The listing builds one solid part. Answer for the finished solid, in the listing's coordinates (mm). A direction names the side the tool comes from. Give positions to 0.01 mm unless a question says otherwise; leave off trailing zeros. Order: outer loops, then holes, each group sorted by start corner. A loop starts at its lowest first (then second) coordinate and runs counter-clockwise, first axis right, second up. Notation, with made-up numbers: (81.25, 53.5) - (138.25, 53.5) arc R11 ccw to (138.25, 67.5) - close; hole circle Ø4 at (39.5, 77.25). An arc over 180 degrees is marked (long way). Answer as a JSON object with one key per item and string values. Group by question number.
Q1. A cutting plane is placed at D-D, the plane x = 0.4. Give the vertices of the cut face in (y, z).
Q2. A cutting plane is placed at B-B, the plane x = 0. Give the vertices of the cut face in (y, z), and give its area (3 significant figures).
Q3. A cutting plane is placed at C-C, the plane z = -1. Give the vertices of the cut face in (x, y), and give its area (3 significant figures).
Q4. A cutting plane is placed at A-A, the plane x = 1.4. Give the vertices of the cut face in (y, z).
Q5. The mould has two halves that part along X. Classify faces 4 (the face through (-0.03, -1.14, -9.09)), 5 (the face through (-0.046, -2.538, -6.086)), 6 (the face through (-2, -3, -3)): released by +X, released by -X, zero draft, split by the parting line, or undercut.
Q6. For faces 1 (the face through (0, -3, -3.4)), 2 (the face through (-0.028, -1.185, -0.722)), 3 (the face through (-0.03, -2.17, -5.71)), determine the directions among +Z, -Z, +X, -X, +Y, -Y from which every point of the face is accessible in a straight line to the end or side of a thin tool.
Q7. Given pin 1 (1 mm diameter, centred on x = 0, y = -3, fed in from +Z); pin 2 (1 mm diameter, centred on x = 0.5, y = -4.5, fed in from -Z); pin 3 (1.5 mm diameter, centred on x = 1, y = -3.5, fed in from -Z), each flat-ended and moving along its own axis, determine where each tip first touches the part or whether it passes through.
Q8. Consider line 1 (Y direction, x = 0.25, z = -2); line 2 (Z direction, x = -1.45, y = -1.9); line 3 (X direction, y = -2.2, z = -7). Determine where each line is inside the solid, lowest interval first.
Autodesk Inventor part; units mm, degrees
ref_plane "YZ Plane" through (0, 0, 0) normal (1, 0, 0) x (0, 1, 0)
ref_plane "XZ Plane" through (0, 0, 0) normal (0, 1, 0) x (-1, 0, 0)
ref_plane "XY Plane" through (0, 0, 0) normal (0, 0, 1) x (1, 0, 0)
sketch "Skizze1" plane through (0, 0, 0) normal (1, 0, 0) x (0, 1, 0)
  line L0 (-1.5214, 0) -> (-5.9349, 0)
  line L1 (-5.9349, 0) -> (-1.5967, -9.3035)
  line L2 (0, -3.2627) -> (-1.5214, 0)
  line L3 (0, -3.2627) -> (-2.7189, -4.5306)
  line L4 (-2.7189, -4.5306) -> (-0.6904, -8.8808)
  line L5 (-0.6904, -8.8808) -> (-1.5967, -9.3035)
  line L6 (0, 1.8607) -> (0, -11.1642)
  point P0 (0, 0)
  dimension "d0" = 65
  dimension "d32" = 1
  dimension "d33" = 3
  dimension "d35" = 3.6
  dimension "d36" = 8.4
extrude "Extrusion1" add sketch "Skizze1" along normal mid plane 4
sketch "Skizze2" plane through (-2, -5.9349, 0) normal (0, 0, 1) x (1, 0, 0)
  line L0 (0, 0) -> (4, 0)
  line L1 (4, 4.4135) -> (4, 0)
  line L2 (4, 4.4135) -> (0, 4.4135)
  line L3 (0, 0) -> (0, 4.4135)
  line L4 (0, 4.3383) -> (0, 0) construction
  point P0 (2, 5.9349)
  point P1 (0, 4.7343)
  point P2 (2, 3.0135)
  dimension "d5" = 2
  dimension "d25" = 1.4
hole "Bohrung1" at (0, -2.9214, 0) direction (0, 0, -1) diameter 1.9 depth 3.4
sketch "Skizze3" plane through (-2, -1.8641, -8.7299) normal (0, -0.9063078, -0.4226183) x (1, 0, 0)
  line L0 (4, 9.6324) -> (4, -0.6329)
  line L1 (0, 9.6324) -> (4, 9.6324)
  line L2 (0, -0.6329) -> (0, 9.6324)
  line L3 (0, -0.6329) -> (4, -0.6329)
  point P0 (2, 1.6324)
  dimension "d26" = 2
  dimension "d29" = 8
hole "Bohrung2" at (0, -2.554, -7.2505) direction (0, 0.9063078, 0.4226183) diameter 2.1 end through all
chamfer "Fase1" distance 1.2 angle 45 1 edges at (0, 0, -3.2627)
fillet "Rundung1" radius 2 1 edges at (0, -0.5071, -2.1751)
properties part number "Ballsensor Platinenwinkel" material "PC/ABS-Kunststoff"
Reply:
{
 "1": {"outline": "(-5.93, 0) - (-2.96, -6.37) - (-2.06, -5.95) - (-2.72, -4.53) - (-1.09, -3.77) - (-0.79, -2.95) arc R2 ccw to (-0.86, -1.42) - (-1.52, 0) - (-2.06, 0) - (-2.06, -3.4) - (-3.78, -3.4) - (-3.78, 0) - close; (-2.14, -8.13) - (-1.6, -9.3) - (-0.69, -8.88) - (-1.24, -7.71) - close"},
 "2": {"outline": "(-5.93, 0) - (-3, -6.3) - (-2.09, -5.88) - (-2.72, -4.53) - (-1.09, -3.77) - (-0.79, -2.95) arc R2 ccw to (-0.86, -1.42) - (-1.52, 0) - (-1.97, 0) - (-1.97, -3.4) - (-3.87, -3.4) - (-3.87, 0) - close; (-2.11, -8.2) - (-1.6, -9.3) - (-0.69, -8.88) - (-1.2, -7.78) - close", "area": "13.6 mm^2"},
 "3": {"outline": "(-2, -5.47) - (2, -5.47) - (2, -1.06) - (-2, -1.06) - close; hole circle Ø1.9 at (0, -2.92)", "area": "14.8 mm^2"},
 "4": {"outline": "(-5.93, 0) - (-1.6, -9.3) - (-0.69, -8.88) - (-2.72, -4.53) - (-1.09, -3.77) - (-0.79, -2.95) arc R2 ccw to (-0.86, -1.42) - (-1.52, 0) - close"},
 "5": {"face 4": "zero draft", "face 5": "undercut", "face 6": "released by -X"},
 "6": {"face 1": "+Z", "face 2": "+Z, +X, -X, +Y", "face 3": "+X, -X, +Y"},
 "7": {"pin 1": "stops at z = -3.4", "pin 2": "stops at z = -4.15", "pin 3": "stops at z = -6.83"},
 "8": {"line 1": "y = -5 to -3.84, -2 to -0.69", "line 2": "z = -8.65 to -6.29, -4.15 to 0", "line 3": "x = -2 to -1.05, 1.05 to 2"}
}
